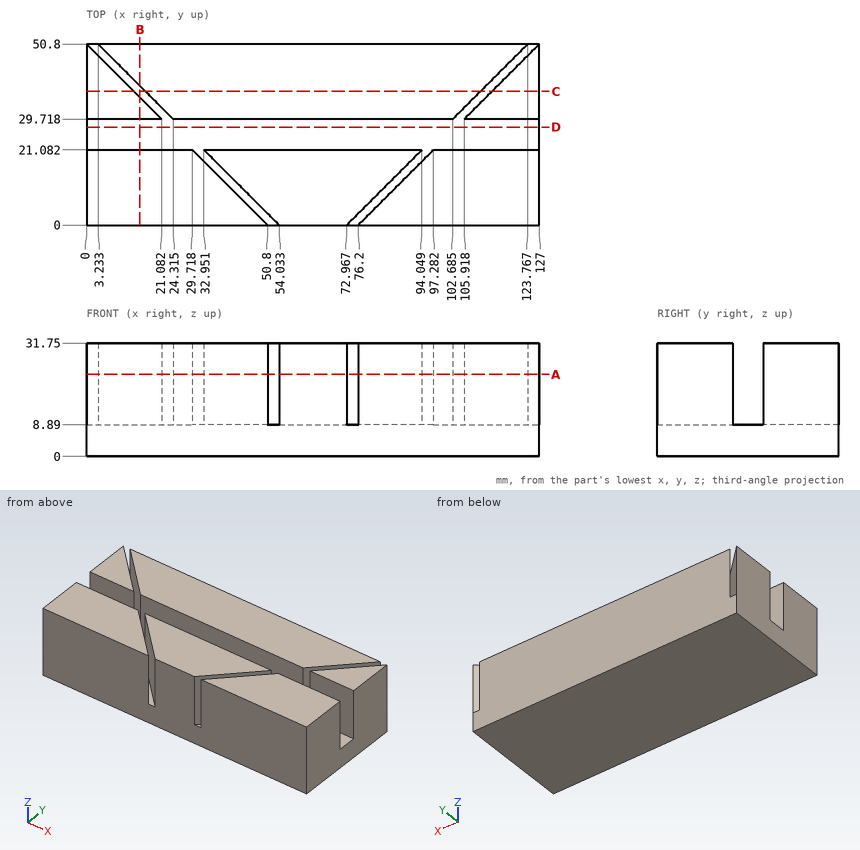
Verification items for this drawing (mm, ordinates from the low corner). Coordinates: 2 decimals unless noted, no trailing zeros. Loops run counter-clockwise (first coordinate to the right, second up) from the corner with the lowest first, then second, coordinate; pieces in that order, holes last. Notation, with made-up numbers: (-12, -8) - (20, -8) arc R26 ccw to (20, 6) - close; hole circle Ø9 at (27, -7.75). An arc over 180 degrees is marked (long way). Answer as a JSON object with one key per item and string values.
(1) Cross-section at A-A, the plane z = 23. Record the boundary of the cut face in (x, y) (3 decimals), then the cut area to 3 significant figures.
Response:
{"outline": "(0, 0) - (50.8, 0) - (29.718, 21.082) - (0, 21.082) - close; (0, 29.718) - (21.082, 29.718) - (0, 50.8) - close; (3.233, 50.8) - (24.315, 29.718) - (102.685, 29.718) - (123.767, 50.8) - close; (32.951, 21.082) - (54.033, 0) - (72.967, 0) - (94.049, 21.082) - close; (76.2, 0) - (127, 0) - (127, 21.082) - (97.282, 21.082) - close; (105.918, 29.718) - (127, 29.718) - (127, 50.8) - close", "area": "5,080 mm²"}
(2) Cross-section at D-D, the plane y = 27.5. Record the boundary of the cut face in (x, z), then the cut area to 3 significant figures.
Response:
{"outline": "(0, 0) - (127, 0) - (127, 8.89) - (0, 8.89) - close", "area": "1,130 mm²"}
(3) Cross-section at C-C, the plane y = 37.5. Record the boundary of the cut face in (x, z).
Response:
{"outline": "(0, 0) - (127, 0) - (127, 31.75) - (113.7, 31.75) - (113.7, 8.89) - (110.47, 8.89) - (110.47, 31.75) - (16.53, 31.75) - (16.53, 8.89) - (13.3, 8.89) - (13.3, 31.75) - (0, 31.75) - close"}
(4) Cross-section at B-B, the plane x = 15. Record the boundary of the cut face in (y, z).
Response:
{"outline": "(0, 0) - (50.8, 0) - (50.8, 31.75) - (39.03, 31.75) - (39.03, 8.89) - (35.8, 8.89) - (35.8, 31.75) - (29.72, 31.75) - (29.72, 8.89) - (21.08, 8.89) - (21.08, 31.75) - (0, 31.75) - close"}
(5) Scan lines: line 1 along Y through (x, z) = (111.5, 16); line 2 along X through (y, z) = (12.5, 9); line 3 along X through (y, z) = (46.5, 29.5). Record each from-to range of solid material in increasing order.
Response:
{"line 1": "y = 0 to 21.08, 29.72 to 35.3, 38.53 to 50.8", "line 2": "x = 0 to 38.3, 41.53 to 85.47, 88.7 to 127", "line 3": "x = 0 to 4.3, 7.53 to 119.47, 122.7 to 127"}
